from build123d import *

# Parameters (mm, degrees)
F0_W     = 88.9
F0_H     = 38.1
F1_DEPTH = 50.8
F2_W     = 12.7
F2_H     = 25.4
F3_DEPTH = 50.801
F4_W     = 25.4
F4_H     = 25.4
F5_DEPTH = 50.801
F6_R     = 6.35
F7_DEPTH = 50.801
F8_W     = 25.4
F8_H     = 50.8
F9_DEPTH = 6.35


with BuildPart() as f1:
    # F0 (on Front) → F1 (new body)
    with BuildSketch(Plane.XZ):
        Rectangle(F0_W, F0_H)
    extrude(amount=F1_DEPTH)

    # F2 (on face) → F3 (cut, through all)
    with BuildSketch(Plane.XZ.offset(50.8)):
        with Locations((-38.1, 6.35)):
            Rectangle(F2_W, F2_H)
    extrude(amount=-F3_DEPTH, mode=Mode.SUBTRACT)

    # F4 (on face) → F5 (cut, through all)
    with BuildSketch(Plane.XZ.offset(50.8)):
        with Locations((31.75, 6.35)):
            Rectangle(F4_W, F4_H)
    extrude(amount=-F5_DEPTH, mode=Mode.SUBTRACT)

    # F6 (on face) → F7 (cut, through all)
    with BuildSketch(Plane.XZ.offset(50.8)):
        with Locations((-4.736888, -6.35)):
            Circle(F6_R)
    extrude(amount=-F7_DEPTH, mode=Mode.SUBTRACT)

    # F8 (on face) → F9 (cut)
    with BuildSketch(Plane.XY.offset(19.05)):
        with Locations((-6.35, -25.4)):
            Rectangle(F8_W, F8_H)
    extrude(amount=-F9_DEPTH, mode=Mode.SUBTRACT)


solid = f1.part
Can you work these out from the model? Positions are in its coordinate system, mm. A direction names the side the tool comes from. Round coordinates to 2 decimals unless told otherwise and drop trailing zeros. Loops run counter-clockwise (first coordinate to the right, second up) from the corner with the lowest first, then second, coordinate; pieces in that order, holes last. Notation, with made-up numbers: (16, -33) - (49, -33) arc R29 ccw to (49, -6) - close; hole circle Ø6 at (-28, 48). An arc over 180 degrees is marked (long way). Answer in a Markdown table with one row per item. Add a question column.
Q1. I want a section at B-B on z = 9. List the corners of the cut face in (x, y) for me, and give its area (3 significant figures).
Q2. I need wall thicknesses on L1, parallel to X at y = -23, z = -6; L2, parallel to X at y = -38, z = 15; L3, parallel to Z at x = 37, y = -6.5. Which ranges of each line are inside material? Lowest first, please.
Q3. I want a section at A-A on y = -38. List the corners of the cut face in (x, z) for me, and give its area (3 significant figures).
Q4. We'd pull the mould along Z, two halves only. Please class faces 1 (the cylindrical face through (1.13, -25.76, -8.78)), 2 (the flat face through (-25, -25, 19.05)), 3 (the flat face through (19.05, -26, 6)): pulls with the +Z half, pulls with the -Z half, needs draft (parallel to the pull), parting line crosses it, or undercut.
Q5. For pin 1 Ø7.5 at (x, y) = (-10, -18.5) entering from +Z; pin 2 Ø4 at (x, y) = (-39.5, -15) entering from +Z; pin 3 Ø5 at (y, z) = (-32.5, 14.5) entering from -X, each with a flat end and sliding along its axis, tell me the tip position at first contact or that it passes through.
Q6. Which directions (+Z, -Z, +X, -X, +Y, -Y) give clear straight access to the entire face, cutting with the end or side of a thin tool? Please do faces 4 (the flat face through (-7, -25, 12.7)), 5 (the flat face through (-31.75, -26, 6)), 6 (the flat face through (32, -26, -6.35)).
Q7. I want a section at C-C on x = 24.5. List the corners of the cut face in (y, z) for me.
A:
| question | item | result |
|---|---|---|
| 1 | outline | (-31.75, -50.8) - (19.05, -50.8) - (19.05, 0) - (-31.75, 0) - close |
| 1 | area | 2,580 mm^2 |
| 2 | L1 | -31.75 to -11.08, 1.6 to 19.05 |
| 2 | L2 | -31.75 to -19.05, 6.35 to 19.05 |
| 2 | L3 | -19.05 to -6.35 |
| 3 | outline | (-44.45, -19.05) - (44.45, -19.05) - (44.45, -6.35) - (19.05, -6.35) - (19.05, 19.05) - (6.35, 19.05) - (6.35, 12.7) - (-19.05, 12.7) - (-19.05, 19.05) - (-31.75, 19.05) - (-31.75, -6.35) - (-44.45, -6.35) - close; hole circle Ø12.7 at (-4.74, -6.35) |
| 3 | area | 2,130 mm^2 |
| 4 | face 1 | undercut |
| 4 | face 2 | pulls with the +Z half |
| 4 | face 3 | needs draft |
| 5 | pin 1 | z = 12.7 |
| 5 | pin 2 | z = -6.35 |
| 5 | pin 3 | x = -31.75 |
| 6 | face 4 | +Z, +Y, -Y |
| 6 | face 5 | +Z, -X, +Y, -Y |
| 6 | face 6 | +Z, +X, +Y, -Y |
| 7 | outline | (-50.8, -19.05) - (0, -19.05) - (0, -6.35) - (-50.8, -6.35) - close |
